Could you check a few things on this model? Use its own coordinates, in mm. Face numbers are marked on the shaded views. A direction names the side the tool comes from. Give positions to 0.01 mm unless a question says otherwise; leave off trailing zeros. Write each question's results on one line, items separated by ' | '. Start each with the question number.
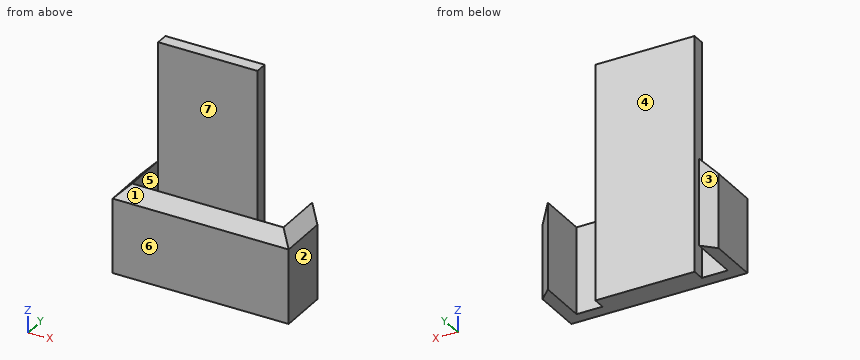
Autodesk Inventor part; units mm, degrees
ref_plane "YZ Plane" through (0, 0, 0) normal (1, 0, 0) x (0, 1, 0)
ref_plane "XZ Plane" through (0, 0, 0) normal (0, 1, 0) x (-1, 0, 0)
ref_plane "XY Plane" through (0, 0, 0) normal (0, 0, 1) x (1, 0, 0)
sketch "스케치1" plane through (0, 0, 0) normal (0, 0, 1) x (1, 0, 0)
  line L0 (0, 5) -> (0, 0)
  line L1 (0, 0) -> (15.1186, 0)
  line L2 (0, 0) -> (14.2, 0)
  line L3 (14.2, 0) -> (14.2, 5)
  line L4 (14.2, 5) -> (13.2, 5)
  line L5 (13.2, 5) -> (13.2, 1)
  line L6 (13.2, 1) -> (1, 1)
  line L7 (1, 1) -> (1, 5)
  line L8 (1, 5) -> (0, 5)
  dimension "t" = 1
  dimension "d1" = 1
  dimension "d2" = 1
  dimension "d3" = 12.2
  dimension "d4" = 4
extrude "돌출1" add sketch "스케치1" along normal blind 7
sketch "스케치2" plane through (1, 1, 0) normal (0, 1, 0) x (1, 0, 0)
  line L0 (12.2, 0) -> (0, 0)
  line L1 (0, 0) -> (0, -7)
  line L2 (12.2, 0) -> (12.2, -7)
  line L3 (10.1, 0) -> (2.1, 0)
  line L4 (2.1, 0) -> (2.1, -19)
  line L5 (2.1, -19) -> (10.1, -19)
  line L6 (10.1, -19) -> (10.1, 0)
  point P0 (-1, 0)
  point P1 (2.1, 0)
  dimension "d7" = 2.1
  dimension "d8" = 19
  dimension "d9" = 2.1
extrude "돌출2" add sketch "스케치2" along normal blind 1
chamfer "모따기1" distance 1 angle 45 5 edges at (14.2, 5, 3.5) (7.1, 0, 7) (0, 5, 3.5) (14.2, 2.5, 7) (0, 2.5, 7)
equation "\"d1\" = t"
equation "\"d2\" = t"
properties part number "_3D 인쇄"
Q1. I'm going to push flat-ended pins straight in: P1, Ø1.7, axis at x = 2, z = 5, coming from the +Y side; P2, Ø6.5, axis at x = 7.5, z = 13.5, coming from the -Y side; P3, Ø2.5, axis at x = 7, z = 5.5, coming from the +Y side. Where does each tip first touch, or does it pass through?
Q2. For the marked faces 5, 6 and 7, which set-ups out of +Z, -Z, +X, -X, +Y, -Y let a thin tool reach every point of the face, with its end or its side?
Q3. Please list where these lines run through material, in increasing order: line 1 (X direction, y = 1.95, z = 2.5); line 2 (X direction, y = 2.95, z = 4.75); line 3 (Y direction, x = 7.5, z = 13.5). Write a range as [from, to].
Q4. If we mould it in two halves opening along X, with no side actions, what happens to the marked faces 1, 2, 3 and 4? For each: pulls with the +X half, pulls with the -X half, needs draft (parallel to the pull), parting line crosses it, or undercut.
Q5. If we section it at A-A (y = 1.65): Count the separate pieces of the cut face and the enclosed holes in it, plus the area to 3 significant figures.
Determined:
1) P1: stops at y = 1 | P2: stops at y = 1 | P3: stops at y = 2
2) face 5: +Z, -Z, +Y | face 6: +Z, -Z, +X, -X, -Y | face 7: +Z, +X, -X, -Y
3) line 1: x = [0, 1], [3.1, 11.1], [13.2, 14.2] | line 2: x = [0, 1], [13.2, 14.2] | line 3: y = [1, 2]
4) face 1: needs draft | face 2: pulls with the +X half | face 3: pulls with the -X half | face 4: undercut
5) separate pieces: 3 | enclosed holes: 0 | area: 165 mm²
